Geometry check sheet. Reference: the model listing, model coordinates, mm. Give positions to 0.01 mm unless a question says otherwise; leave off trailing zeros. Loops run counter-clockwise (first coordinate to the right, second up) from the corner with the lowest first, then second, coordinate; pieces in that order, holes last.
1. Cross-section at A-A, the plane x = 0. Record the cut outline in (y, z), plus the area to 3 significant figures.
2. Release check for a two-part mould opening along X. For faces 1 (the flat face through (-2.39, 9.86, 1.36)), 2 (the cylindrical face through (-0.37, 9.86, -1.66)), 3 (the flat face through (2.37, 9.863, 1.394)) record: +X half, -X half, draft (parallel to the pull), parting line (faces both ways), or undercut.
3. Material ranges on L1, parallel to Z at x = 0, y = 5.5; L2, parallel to X at y = 18, z = 1.2; L3, parallel to X at y = 19, z = -0.7, recorded low to high.
4. Cross-section at B-B, the plane y = 4. Record the cut outline in (x, z), plus the area to 3 significant figures.
from build123d import *

# Parameters (mm, degrees)
BOSS_EXTRUDE1_DEPTH      = 20
M3_CLEARANCE_HOLE1_D     = 3.4
M3_CLEARANCE_HOLE1_DEPTH = 20
M3_CLEARANCE_HOLE1_TIP   = 1.021463052


with BuildPart() as part:
    # Sketch1 → Boss-Extrude1 (new body)
    with BuildSketch(Plane(origin=(0, 0, 0), x_dir=(1, 0, 0), z_dir=(0, 1, 0))):
        Polygon((3.175426481, 0), (1.58771324, 2.75), (-1.58771324, 2.75), (-3.175426481, 0), (-1.58771324, -2.75), (1.58771324, -2.75), align=None)
    extrude(amount=BOSS_EXTRUDE1_DEPTH)

    # M3 Clearance Hole1
    with Locations(Plane(origin=(0, 20, 0), x_dir=(-1, 0, 0), z_dir=(0, 1, 0))):
        with Locations((0, 0)):
            Hole(M3_CLEARANCE_HOLE1_D / 2, depth=M3_CLEARANCE_HOLE1_DEPTH)
            with Locations((0, 0, -(M3_CLEARANCE_HOLE1_DEPTH + M3_CLEARANCE_HOLE1_TIP / 2))):  # 118° drill point
                Cone(0, M3_CLEARANCE_HOLE1_D / 2, M3_CLEARANCE_HOLE1_TIP, mode=Mode.SUBTRACT)

    # Sketch4 → Cut-Revolve1 (revolve, cut)
    with BuildSketch(Plane.XY, mode=Mode.PRIVATE) as cut_revolve1_sk:
        with BuildLine():
            Line((-2.175426481, 20), (-3.175426481, 20))
            Line((-3.175426481, 20), (-3.175426481, 19))
            ThreePointArc((-3.175426481, 19), (-2.882533262, 19.707106781), (-2.175426481, 20))
        make_face()
        with BuildLine():
            Line((-3.175426481, 1), (-3.175426481, 0))
            Line((-3.175426481, 0), (-2.175426481, 0))
            ThreePointArc((-2.175426481, 0), (-2.882533262, 0.292893219), (-3.175426481, 1))
        make_face()
    revolve(cut_revolve1_sk.sketch.rotate(Axis((0, 20, 0), (0, -1, 0)), 270), axis=Axis((0, 20, 0), (0, -1, 0)), mode=Mode.SUBTRACT)


solid = part.part
Result:
1. outline: (0, -2.18) arc R1 ccw to (0.18, -2.75) - (19.82, -2.75) arc R1 ccw to (20, -2.18) - (20, -1.7) - (0, -1.7) - close; (0, 1.7) - (20, 1.7) - (20, 2.18) arc R1 ccw to (19.82, 2.75) - (0.18, 2.75) arc R1 ccw to (0, 2.18) - close
1. area: 41.9 mm2
2. face 1: -X half
2. face 2: undercut
2. face 3: +X half
3. L1: z = -2.75 to -1.7, 1.7 to 2.75
3. L2: x = -2.48 to -1.2, 1.2 to 2.48
3. L3: x = -2.77 to -1.55, 1.55 to 2.77
4. outline: (-3.18, 0) - (-1.59, -2.75) - (1.59, -2.75) - (3.18, 0) - (1.59, 2.75) - (-1.59, 2.75) - close; hole circle Ø3.4 at (0, 0)
4. area: 17.1 mm2
